Read the model definition and answer for the solid it produces. Units are mm, in the model's axes. Round coordinates to 2 decimals unless told otherwise and drop trailing zeros. Loops run counter-clockwise (first coordinate to the right, second up) from the corner with the lowest first, then second, coordinate; pieces in that order, holes last. Notation, with made-up numbers: (43.5, -36) -> (75.5, -36) arc R15 cw to (75.5, -19) -> close; hole circle Ø3 at (-24, 33). An arc over 180 degrees is marked (long way). Put each result on its own line as item: value.
from build123d import *

# Parameters (mm, degrees)
SKETCH1_R           = 15
BOSS_EXTRUDE1_DEPTH = 17
SKETCH2_R           = 1
CUT_EXTRUDE1_DEPTH  = 17
FILLET3_R           = 2.5


with BuildPart() as part:
    # Sketch1 → Boss-Extrude1 (new body)
    with BuildSketch(Plane.XY):
        Circle(SKETCH1_R)
    extrude(amount=BOSS_EXTRUDE1_DEPTH)

    # Sketch2 → Cut-Extrude1 (cut)
    with BuildSketch(Plane(origin=(0, 0, 0), x_dir=(-1, 0, 0), z_dir=(0, 0, -1))):
        Circle(SKETCH2_R)
    extrude(amount=-CUT_EXTRUDE1_DEPTH, mode=Mode.SUBTRACT)

    # Fillet3
    fillet3_edges = [part.edges().sort_by_distance(p)[0] for p in [
        (-15, 0, 0),
        (-15, 0, 17),
        (1, 0, 17),
    ]]
    fillet(fillet3_edges, radius=FILLET3_R)


solid = part.part
Item 1: For a pull along Y with two mould halves and no side action, classify faces 1 (the flat face through (3, -3, 17)), 2 (the cylindrical face through (0, -1, 7)), 3 (the cylindrical face through (-14.985, 0.66, 8.416)) as pulls with the +Y half, pulls with the -Y half, needs draft (parallel to the pull), parting line crosses it, or undercut.
Derived:
face 1: needs draft
face 2: undercut
face 3: parting line crosses it
Item 2: The part is cut by section C-C (z = 12.5). Determine the outline of the cut face in (x, y), then the cut area to 3 significant figures.
Derived:
outline: circle Ø30 at (0, 0); hole circle Ø2 at (0, 0)
area: 704 mm^2
Item 3: Find the intervals of material crossed by line 1 along Y through (x, z) = (0, 5); line 2 along X through (y, z) = (-3, 3.5); line 3 along Y through (x, z) = (8, 15), in increasing order.
Derived:
line 1: y = -15 to -1, 1 to 15
line 2: x = -14.7 to 14.7
line 3: y = -12.63 to 12.63
Item 4: Flat-ended cylindrical pins translate along their axes: pin 1 Ø10 at (x, z) = (-8, 9.5) entering from -Y; pin 2 Ø5 at (x, z) = (11, 7.5) entering from +Y; pin 3 Ø2 at (x, z) = (-5.5, 14) entering from -Y. Find the tip coordinate at first contact, or state that the pin passes through.
Derived:
pin 1: stops at y = -14.7
pin 2: stops at y = 12.36
pin 3: stops at y = -14.31
Item 5: The part is cut by section A-A (x = 0). Determine the outline of the cut face in (y, z), then the cut area to 3 significant figures.
Derived:
outline: (-15, 2.5) arc R2.5 ccw to (-12.5, 0) -> (-1, 0) -> (-1, 14.5) arc R2.5 ccw to (-3.5, 17) -> (-12.5, 17) arc R2.5 ccw to (-15, 14.5) -> close; (1, 0) -> (12.5, 0) arc R2.5 ccw to (15, 2.5) -> (15, 14.5) arc R2.5 ccw to (12.5, 17) -> (3.5, 17) arc R2.5 ccw to (1, 14.5) -> close
area: 468 mm^2
